Check sheet for the modelled part. Datum: model origin and axes. Units: mm. A direction names the side the tool comes from. Round coordinates to 2 decimals unless told otherwise and drop trailing zeros. Order: outer loops, then holes, each group sorted by start corner. A loop starts at its lowest first (then second) coordinate and runs counter-clockwise, first axis right, second up. Notation, with made-up numbers: (73, -3) -> (93, -3) arc R33 cw to (93, 29) -> close; hole circle Ø11 at (63.25, -31.75). An arc over 180 degrees is marked (long way). Answer in a Markdown table with one row per item.
```python
from build123d import *

# Parameters (mm, degrees)
EXTRUDE_1_DEPTH          = 15.25
CUT_EXTRUDE_1_DEPTH      = 26.550195694
CUT_EXTRUDE_1_DEPTH_BACK = 26.550195694
SKETCH_3_W               = 8.238165393
SKETCH_3_H               = 6.875
SKETCH_4_R               = 2
CUT_EXTRUDE_2_DEPTH      = 32.279236324
PATTERN_LINEAR_1_COUNT   = 2
PATTERN_LINEAR_1_PITCH   = 14


with BuildPart() as part:
    # 草图1 → 凸台-拉伸1 (new, symmetric)
    with BuildSketch(Plane.XY):
        with BuildLine():
            Line((17.464816242, 0), (4, 0))
            ThreePointArc((4, 0), (-2.371533507, 3.221153338), (-1.187914412, -3.819536536))
            Line((-1.187914412, -3.819536536), (1, -4.5))
            Line((1, -4.5), (20, -4.5))
            Line((20, -4.5), (20, -3.302775638))
            ThreePointArc((20, -3.302775638), (19.957092026, -3.012991489), (19.832050294, -2.748075442))
            Line((19.832050294, -2.748075442), (18.296866536, -0.445299804))
            ThreePointArc((18.296866536, -0.445299804), (17.936674167, -0.118325401), (17.464816242, 0))
        make_face()
    extrude(amount=EXTRUDE_1_DEPTH, both=True)

    # 草图3 → 切除-拉伸1 (cut, two sides: drawn at the far end of the back side and taken through both)
    with BuildSketch(Plane(origin=(0, 0, 0), x_dir=(1, 0, 0), z_dir=(0, 1, 0)).offset(-CUT_EXTRUDE_1_DEPTH_BACK)):
        with Locations((0.119082697, -11.8125)):
            Rectangle(SKETCH_3_W, SKETCH_3_H)
        with Locations((0.119082697, 3.9475)):
            Rectangle(SKETCH_3_W, SKETCH_3_H)
    extrude(amount=CUT_EXTRUDE_1_DEPTH + CUT_EXTRUDE_1_DEPTH_BACK, mode=Mode.SUBTRACT)

    # 草图4 → 切除-拉伸2 (cut, through all)
    with BuildSketch(Plane.XY.offset(8.375)):
        Circle(SKETCH_4_R)
    extrude(amount=-CUT_EXTRUDE_2_DEPTH, mode=Mode.SUBTRACT)

    # 草图5 → 切除-旋转1 (revolve, cut)
    with BuildSketch(Plane.XY.offset(7), mode=Mode.PRIVATE) as cut_revolve_1_sk:
        Polygon((10, -4.5), (10, 0), (14.4, 0), (14.4, -0.5), (12.5, -2), (12.5, -4.5), align=None)
    cut_revolve_1 = revolve(cut_revolve_1_sk.sketch.rotate(Axis((10, -4.5, 7), (0, 1, 0)), 90), axis=Axis((10, -4.5, 7), (0, 1, 0)), mode=Mode.SUBTRACT)

    # 阵列(线性)1: 切除-旋转1 ×2
    with Locations(*[(0, 0, -i * PATTERN_LINEAR_1_PITCH) for i in range(1, PATTERN_LINEAR_1_COUNT)]):
        add(cut_revolve_1, mode=Mode.SUBTRACT)


solid = part.part
```
(1) Scan lines: probe 1 along X at (y, z) = (-1.5, 5); probe 2 along Z at (x, y) = (3.5, -1) (3 decimals); probe 3 along Y at (x, z) = (17.5, -12.5). Record each from-to range of solid material in increasing order. Write a range as from..to.
Solutions:
| item | result |
|---|---|
| probe 1 | -3.71..-1.32, 1.32..7.59, 12.41..19 |
| probe 2 | -15.25..-7.385, -0.51..8.375 |
| probe 3 | -4.5..0 |
(2) Draft check along Z on faces 1 (the conical face through (9.2, -1.9, -9.5)), 2 (the flat face through (4.238, -2, 12)), 3 (the flat face through (4.238, -2, -4)), 4 (the flat face through (12, -2, 15.25)). Enter one of: pulls with the +Z half, pulls with the -Z half, needs draft (parallel to the pull), parting line crosses it, or undercut.
Solutions:
| item | result |
|---|---|
| face 1 | undercut |
| face 2 | needs draft |
| face 3 | undercut |
| face 4 | pulls with the +Z half |
(3) Section check C-C on x = 10. Record the boundary of the cut face in (y, z).
Solutions:
| item | result |
|---|---|
| outline | (-4.5, -15.25) -> (0, -15.25) -> (0, -11.4) -> (-0.5, -11.4) -> (-2, -9.5) -> (-4.5, -9.5) -> close; (-4.5, -4.5) -> (-2, -4.5) -> (-0.5, -2.6) -> (0, -2.6) -> (0, 2.6) -> (-0.5, 2.6) -> (-2, 4.5) -> (-4.5, 4.5) -> close; (-4.5, 9.5) -> (-2, 9.5) -> (-0.5, 11.4) -> (0, 11.4) -> (0, 15.25) -> (-4.5, 15.25) -> close |
(4) Tool access check on faces 5 (the flat face through (11, 0, 0)), 6 (the cylindrical face through (8.678, -0.254, 2.803)), 7 (the flat face through (2, -1, -7.385)), 8 (the flat face through (2, -1, 8.375)). Record the directions out of +Z, -Z, +X, -X, +Y, -Y that give a thin tool (end or side, any length) a straight path to the whole face; none if there is none.
Solutions:
| item | result |
|---|---|
| face 5 | +Z, -Z, +X, +Y |
| face 6 | +Y |
| face 7 | -X, +Y, -Y |
| face 8 | +Z, -X, +Y, -Y |
(5) Section check D-D on y = 0.5. Give the number of separate pieces and of enclosed holes in the cut face, plus the area to 3 significant figures.
Solutions:
| item | result |
|---|---|
| separate pieces | 4 |
| enclosed holes | 0 |
| area | 68.1 mm^2 |
(6) Section check B-B on z = -7. Record the boundary of the cut face in (x, y).
Solutions:
| item | result |
|---|---|
| outline | (4.24, -4.5) -> (7.5, -4.5) -> (7.5, -2) -> (5.6, -0.5) -> (5.6, 0) -> (4.24, 0) -> close; (12.5, -4.5) -> (20, -4.5) -> (20, -3.3) arc R1 ccw to (19.83, -2.75) -> (18.3, -0.45) arc R1 ccw to (17.46, 0) -> (14.4, 0) -> (14.4, -0.5) -> (12.5, -2) -> close |
(7) Section check A-A on z = 7. Record the boundary of the cut face in (x, y).
Solutions:
| item | result |
|---|---|
| outline | (-1.19, -3.82) -> (1, -4.5) -> (7.5, -4.5) -> (7.5, -2) -> (5.6, -0.5) -> (5.6, 0) -> (4, 0) arc R4 ccw (long way) to start; (12.5, -4.5) -> (20, -4.5) -> (20, -3.3) arc R1 ccw to (19.83, -2.75) -> (18.3, -0.45) arc R1 ccw to (17.46, 0) -> (14.4, 0) -> (14.4, -0.5) -> (12.5, -2) -> close; hole circle Ø4 at (0, 0) |
(8) Depth check by flat-ended pin: pin 1 Ø6.5 at (x, z) = (10.5, -1) entering from +Y; pin 2 Ø3 at (y, z) = (2.5, -10.5) entering from -X; pin 3 Ø4 at (x, y) = (1, 1) entering from +Z (3 decimals); pin 4 Ø3 at (x, y) = (0, 0) entering from +Z. Enter the tip coordinate at first touch or a pass-through.
Solutions:
| item | result |
|---|---|
| pin 1 | y = 0 |
| pin 2 | x = -3.87 |
| pin 3 | z = 8.375 |
| pin 4 | through |
